Geometry: see drawing. Coordinates: mm, zero at the bounding-box minimum. A direction names the side the tool comes from. Give positions to 0.01 mm unless a question says otherwise; leave off trailing zeros. Loops run counter-clockwise (first coordinate to the right, second up) from the corner with the lowest first, then second, coordinate; pieces in that order, holes last. Notation, with made-up numbers: (-16, 0.25) - (10, 0.25) arc R32 cw to (10, 27.25) - close; hole circle Ø6 at (9, 29.5). An arc over 180 degrees is marked (long way). One line per question, with ' | ' between items. Start each with the question number.
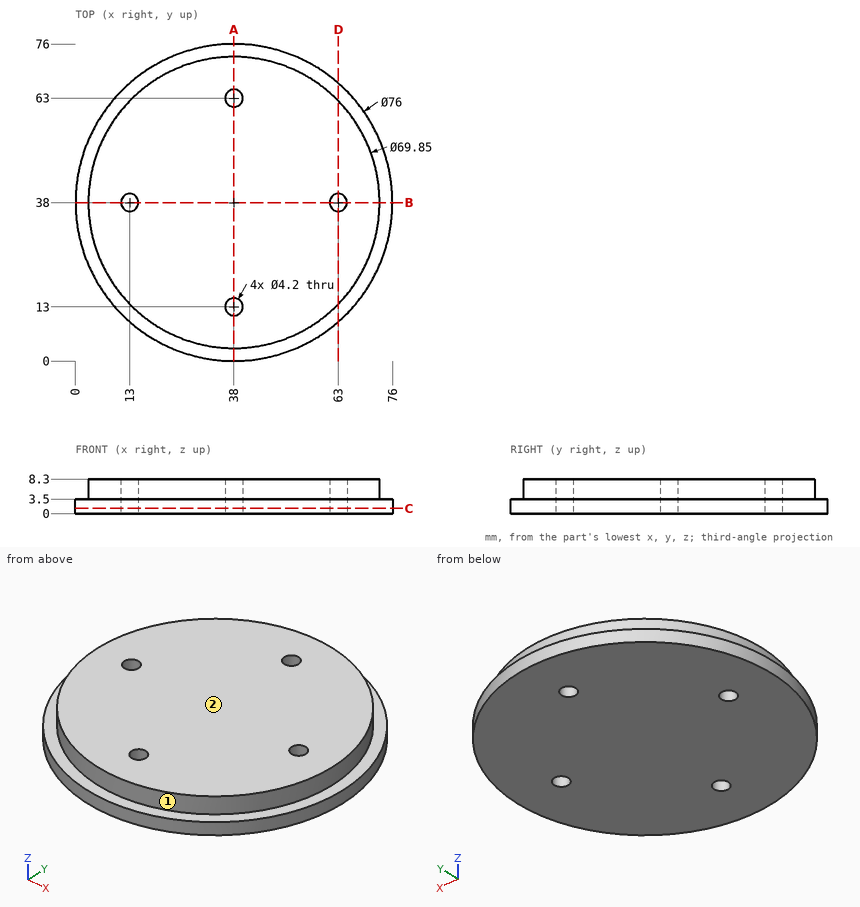
Q1. First-contact query: pin 1 (1.5 mm diameter, centred on x = 41.5, z = 2, fed in from +Y); pin 2 (4 mm diameter, centred on x = 47.5, z = 3, fed in from -Y); pin 3 (4 mm diameter, centred on x = 38, y = 63, fed in from -Z); pin 4 (1 mm diameter, centred on x = 59.5, z = 5.5, fed in from +Y). Flat tips, straight axial feed; report the tip coordinate or a pass-through.
Q2. Line query: L1, parallel to Y at x = 38, z = 3.25; L2, parallel to Y at x = 39, z = 1.5; L3, parallel to Y at x = 16, z = 4.75. Output: solid intervals per line, ascending. Write a range as from..to.
Q3. Section D-D, the plane x = 63. Output: boundary loops of the cut face in (y, z).
Q4. Section A-A, the plane x = 38. Output: boundary loops of the cut face in (y, z) (3 decimals).
Q5. Section C-C, the plane z = 1.25. Output: boundary loops of the cut face in (x, y), plus the area to 3 significant figures.
Q6. Access query for the marked faces 1 and 2. Directions: +Z, -Z, +X, -X, +Y, -Y. A direction counts if a zero-diameter tool reaches every point of the face in a straight line with its end or side. Return the directions, or none.
Solved:
1) pin 1: stops at y = 75.9 | pin 2: stops at y = 0.75 | pin 3: passes through | pin 4: stops at y = 65.91
2) L1: y = 0..10.9, 15.1..60.9, 65.1..76 | L2: y = 0.01..11.15, 14.85..61.15, 64.85..75.99 | L3: y = 10.88..65.12
3) outline: (9.38, 0) - (35.9, 0) - (35.9, 8.3) - (13.61, 8.3) - (13.61, 3.5) - (9.38, 3.5) - close; (40.1, 0) - (66.62, 0) - (66.62, 3.5) - (62.39, 3.5) - (62.39, 8.3) - (40.1, 8.3) - close
4) outline: (0, 0) - (10.9, 0) - (10.9, 8.3) - (3.075, 8.3) - (3.075, 3.5) - (0, 3.5) - close; (15.1, 0) - (60.9, 0) - (60.9, 8.3) - (15.1, 8.3) - close; (65.1, 0) - (76, 0) - (76, 3.5) - (72.925, 3.5) - (72.925, 8.3) - (65.1, 8.3) - close
5) outline: circle Ø76 at (38, 38); hole circle Ø4.2 at (13, 38); hole circle Ø4.2 at (38, 13); hole circle Ø4.2 at (38, 63); hole circle Ø4.2 at (63, 38) | area: 4,480 mm²
6) face 1: +Z | face 2: +Z, +X, -X, +Y, -Y
